Part model, mm, in its own coordinate system. Round coordinates to 2 decimals unless told otherwise and drop trailing zeros. Write each loop counter-clockwise with the first axis right and the second up, starting at its lowest first coordinate (ties: lowest second). Pieces come first, ordered by that corner, then holes. Notation, with made-up numbers: M -24,54.5 L -12,54.5 A5 cw -12,62.5 Z; hole C 53.25,43 d10. An arc over 180 degrees is marked long. One line per question, with ' | ' between items. Start each with the question number.
1) Saw through at C-C (z = -4). List the corners of the cut face in (x, y).
2) Drop flat-ended pins along their axis: pin 1 Ø2 at (x, z) = (0.5, 2.5) entering from -Y; pin 2 Ø1.5 at (x, z) = (-2, 6) entering from -Y; pin 3 Ø0.8 at (x, z) = (-1, 6.5) entering from +Y; pin 4 Ø0.6 at (y, z) = (-0.5, 4.5) entering from +X. Give the stop position or say it passes through.
3) Wall check: probe 1 along X at (y, z) = (-0.15, 5.5); probe 2 along Z at (x, y) = (5.5, 0.6); probe 3 along Y at (x, z) = (-1.25, -4). Give the ranges that are in metal, low to high. Write a range as [from, to].
4) Saw through at B-B (x = 1.5). List the corners of the cut face in (y, z).
5) Saw through at A-A (z = 7.5). List the corners of the cut face in (x, y), plus the area to 3 significant figures.
6) Saw through at D-D (x = -0.25). List the corners of the cut face in (y, z), plus the area to 3 significant figures.
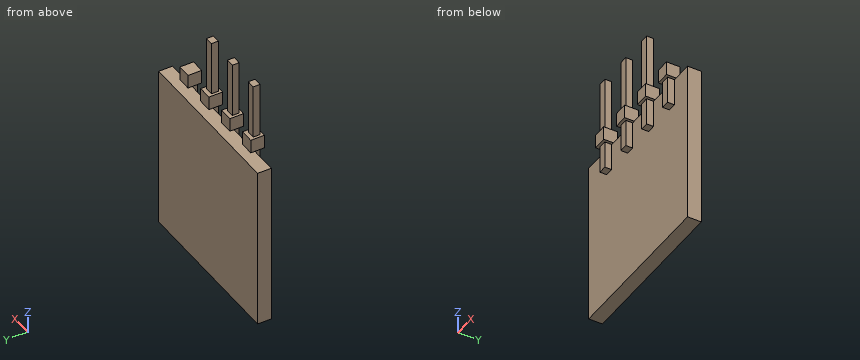
```python
from build123d import *

# Parameters (mm, degrees)
SKETCH1_W           = 12
SKETCH1_H           = 12
BOSS_EXTRUDE1_DEPTH = 1
SKETCH2_W           = 0.6
SKETCH2_H           = 0.5
BOSS_EXTRUDE2_DEPTH = 5
SKETCH2_3_W         = 0.6
SKETCH2_3_H         = 0.5
BOSS_EXTRUDE3_DEPTH = 2
LPATTERN2_COUNT     = 4
LPATTERN2_PITCH     = 2.54
LPATTERN3_COUNT     = 3
LPATTERN3_PITCH     = 2.54
SKETCH3_W           = 1
SKETCH3_H           = 1
BOSS_EXTRUDE4_DEPTH = 1
LPATTERN4_COUNT     = 4
LPATTERN4_PITCH     = 2.54


with BuildPart() as part:
    # Sketch1 → Boss-Extrude1 (new body)
    with BuildSketch(Plane(origin=(0, 0, 0), x_dir=(1, 0, 0), z_dir=(0, 1, 0))):
        Rectangle(SKETCH1_W, SKETCH1_H)
    extrude(amount=BOSS_EXTRUDE1_DEPTH)



with BuildPart() as body_2:
    # Sketch2 → Boss-Extrude2 (new body)
    with BuildSketch(Plane.XY.offset(6)):
        with Locations((-3.51, -0.25)):
            Rectangle(SKETCH2_W, SKETCH2_H)
    boss_extrude2 = extrude(amount=BOSS_EXTRUDE2_DEPTH)


with BuildPart() as part_1:
    add(part.part)

    add(body_2.part)  # Boss-Extrude3 merges body 2
    # Sketch2<3> → Boss-Extrude3 (add)
    with BuildSketch(Plane.XY.offset(6)):
        with Locations((-3.51, -0.25)):
            Rectangle(SKETCH2_3_W, SKETCH2_3_H)
    boss_extrude3 = extrude(amount=-BOSS_EXTRUDE3_DEPTH)

    # LPattern2: Boss-Extrude3 ×4
    with Locations(*[(i * LPATTERN2_PITCH, 0, 0) for i in range(1, LPATTERN2_COUNT)]):
        add(boss_extrude3)

    # LPattern3: Boss-Extrude2 ×3
    with Locations(*[(i * LPATTERN3_PITCH, 0, 0) for i in range(1, LPATTERN3_COUNT)]):
        add(boss_extrude2)

    # Sketch3 → Boss-Extrude4 (add)
    with BuildSketch(Plane.XY.offset(6)):
        with Locations((4.11, -0.2)):
            Rectangle(SKETCH3_W, SKETCH3_H)
    boss_extrude4 = extrude(amount=BOSS_EXTRUDE4_DEPTH)

    # LPattern4: Boss-Extrude4 ×4
    with Locations(*[(-i * LPATTERN4_PITCH, 0, 0) for i in range(1, LPATTERN4_COUNT)]):
        add(boss_extrude4)


solid = part_1.part
```
Answer key:
1) outline: M -6,0 L 6,0 L 6,1 L -6,1 Z
2) pin 1: stops at y = 0 | pin 2: stops at y = -0.7 | pin 3: stops at y = 0.3 | pin 4: stops at x = 4.41
3) probe 1: x = [-3.81, -3.21], [-1.27, -0.67], [1.27, 1.87], [3.81, 4.41] | probe 2: z = [-6, 6] | probe 3: y = [0, 1]
4) outline: M -0.7,6 L -0.5,6 L -0.5,4 L 0,4 L 0,-6 L 1,-6 L 1,6 L 0.3,6 L 0.3,7 L 0,7 L 0,11 L -0.5,11 L -0.5,7 L -0.7,7 Z
5) outline: M -3.81,-0.5 L -3.21,-0.5 L -3.21,0 L -3.81,0 Z; M -1.27,-0.5 L -0.67,-0.5 L -0.67,0 L -1.27,0 Z; M 1.27,-0.5 L 1.87,-0.5 L 1.87,0 L 1.27,0 Z | area: 0.900 mm2
6) outline: M 0,-6 L 1,-6 L 1,6 L 0,6 Z | area: 12.0 mm2
